Geometry: final body of the model. Coordinates: model frame, mm. A direction names the side the tool comes from. Coordinates: 2 decimals unless noted, no trailing zeros. Loops run counter-clockwise (first coordinate to the right, second up) from the corner with the lowest first, then second, coordinate; pieces in that order, holes last. Notation, with made-up numbers: (87, 8) - (98, 8) arc R16 ccw to (98, 16) - close; hole circle Ø11 at (70.5, 55.5). An arc over 180 degrees is marked (long way). Return JSON: item names as keys, results as strings.
from build123d import *

# Parameters (mm, degrees)
SKETCH10_W                   = 276.86
SKETCH10_H                   = 12.7
BASE_FLANGE1_DEPTH           = 1
EDGE_FLANGE1_STRIP_W         = 9.08
EDGE_FLANGE1_STRIP_H         = 1
EDGE_FLANGE1_STRIP_CUT_DEPTH = 276.86
EDGE_FLANGE1_DEPTH           = 276.86
EDGE_FLANGE2_STRIP_W         = 9.08
EDGE_FLANGE2_STRIP_H         = 1
EDGE_FLANGE2_STRIP_CUT_DEPTH = 276.86
EDGE_FLANGE2_DEPTH           = 276.86
EDGE_FLANGE3_STRIP_W         = 9.08
EDGE_FLANGE3_STRIP_H         = 1
EDGE_FLANGE3_STRIP_CUT_DEPTH = 5.62
EDGE_FLANGE3_DEPTH           = 5.62


# Sheet-metal steps are written as plain solids
with BuildPart() as part:
    # Sketch10 → Base-Flange1 (new body)
    with BuildSketch(Plane(origin=(0, 0, 0), x_dir=(1, 0, 0), z_dir=(0, 1, 0))):
        Rectangle(SKETCH10_W, SKETCH10_H)
    extrude(amount=-BASE_FLANGE1_DEPTH)

    # Edge-Flange1 strip (across the edge) → Edge-Flange1 strip cut (cut)
    with BuildSketch(Plane(origin=(138.43, 0, -6.35), x_dir=(0, 0, 1), z_dir=(-1, 0, 0))):
        with Locations((-1, -0.5)):
            Rectangle(EDGE_FLANGE1_STRIP_W, EDGE_FLANGE1_STRIP_H)
    extrude(amount=EDGE_FLANGE1_STRIP_CUT_DEPTH, mode=Mode.SUBTRACT)

    # Edge-Flange1 section (across the edge) → Edge-Flange1 (add)
    with BuildSketch(Plane(origin=(138.43, 0, -6.35), x_dir=(0, 0, 1), z_dir=(-1, 0, 0))):
        with BuildLine():
            Line((0, 2.54), (0, 11.7))
            Line((0, 11.7), (1, 11.7))
            Line((1, 11.7), (1, 2.54))
            ThreePointArc((1, 2.54), (1.743948776, 0.743948776), (3.54, 0))
            Line((3.54, 0), (3.54, -1))
            ThreePointArc((3.54, -1), (1.036841995, 0.036841995), (0, 2.54))
        make_face()
    extrude(amount=EDGE_FLANGE1_DEPTH)

    # Edge-Flange2 strip (across the edge) → Edge-Flange2 strip cut (cut)
    with BuildSketch(Plane(origin=(-138.43, 0, 6.35), x_dir=(0, 0, -1), z_dir=(1, 0, 0))):
        with Locations((-1, -0.5)):
            Rectangle(EDGE_FLANGE2_STRIP_W, EDGE_FLANGE2_STRIP_H)
    extrude(amount=EDGE_FLANGE2_STRIP_CUT_DEPTH, mode=Mode.SUBTRACT)

    # Edge-Flange2 section (across the edge) → Edge-Flange2 (add)
    with BuildSketch(Plane(origin=(-138.43, 0, 6.35), x_dir=(0, 0, -1), z_dir=(1, 0, 0))):
        with BuildLine():
            Line((0, 2.54), (0, 11.7))
            Line((0, 11.7), (1, 11.7))
            Line((1, 11.7), (1, 2.54))
            ThreePointArc((1, 2.54), (1.743948776, 0.743948776), (3.54, 0))
            Line((3.54, 0), (3.54, -1))
            ThreePointArc((3.54, -1), (1.036841995, 0.036841995), (0, 2.54))
        make_face()
    extrude(amount=EDGE_FLANGE2_DEPTH)

    # Edge-Flange3 strip (across the edge) → Edge-Flange3 strip cut (cut)
    with BuildSketch(Plane(origin=(-138.43, 0, -2.81), x_dir=(1, 0, 0), z_dir=(0, 0, 1))):
        with Locations((-1, -0.5)):
            Rectangle(EDGE_FLANGE3_STRIP_W, EDGE_FLANGE3_STRIP_H)
    extrude(amount=EDGE_FLANGE3_STRIP_CUT_DEPTH, mode=Mode.SUBTRACT)

    # Edge-Flange3 section (across the edge) → Edge-Flange3 (add)
    with BuildSketch(Plane(origin=(-138.43, 0, -2.81), x_dir=(1, 0, 0), z_dir=(0, 0, 1))):
        with BuildLine():
            Line((0, 2.54), (0, 11.7))
            Line((0, 11.7), (1, 11.7))
            Line((1, 11.7), (1, 2.54))
            ThreePointArc((1, 2.54), (1.743948776, 0.743948776), (3.54, 0))
            Line((3.54, 0), (3.54, -1))
            ThreePointArc((3.54, -1), (1.036841995, 0.036841995), (0, 2.54))
        make_face()
    extrude(amount=EDGE_FLANGE3_DEPTH)


solid = part.part
Item 1: Mould query, pull axis Z, two halves, no side actions, for faces 1 (the face through (-2, 7, 6.35)), 2 (the face through (-2, 7, 5.35)), 3 (the face through (0, -1, 0)). Classes: +Z half, -Z half, draft (parallel to the pull), parting line (faces both ways), or undercut.
Worked out:
{"face 1": "+Z half", "face 2": "undercut", "face 3": "draft"}
Item 2: Section query B-B, the plane x = 20. Return loops of the section in (y, z), and give its area (3 significant figures).
Worked out:
{"outline": "(-1, -2.81) arc R3.54 ccw to (2.54, -6.35) - (11.7, -6.35) - (11.7, -5.35) - (2.54, -5.35) arc R2.54 cw to (0, -2.81) - (0, 2.81) arc R2.54 cw to (2.54, 5.35) - (11.7, 5.35) - (11.7, 6.35) - (2.54, 6.35) arc R3.54 ccw to (-1, 2.81) - close", "area": "33.5 mm^2"}
Item 3: Reachability of faces 4 (the face through (2, 7, -5.35)), 5 (the face through (-137.43, 7, 0)), 6 (the face through (2, 7, -6.35)) from +Z, -Z, +X, -X, +Y, -Y: full face, straight path, thin tool, end or side. Return the list, or none.
Worked out:
{"face 4": "+X, -X, +Y", "face 5": "+X, +Y", "face 6": "-Z, +X, -X, +Y, -Y"}
Item 4: Section query A-A, the plane y = 7.25. Return loops of the section in (x, z), and give its area (3 significant figures).
Worked out:
{"outline": "(-138.43, -6.35) - (138.43, -6.35) - (138.43, -5.35) - (-138.43, -5.35) - close; (-138.43, -2.81) - (-137.43, -2.81) - (-137.43, 2.81) - (-138.43, 2.81) - close; (-138.43, 5.35) - (138.43, 5.35) - (138.43, 6.35) - (-138.43, 6.35) - close", "area": "559 mm^2"}
Item 5: First-contact query: pin 1 Ø3 at (x, z) = (18, 1.5) entering from +Y; pin 2 Ø2 at (y, z) = (5.5, 0.5) entering from +X; pin 3 Ø0.8 at (x, y) = (-136, -0.5) entering from +Z. Flat tips, straight axial feed; report the tip coordinate or a pass-through.
Worked out:
{"pin 1": "y = 0.01", "pin 2": "x = -137.43", "pin 3": "z = 5.17"}
Item 6: Ray query, probe 1 along Z at (x, y) = (105, 9); probe 2 along Y at (x, z) = (44, 2.25); probe 3 along Z at (x, y) = (39, 1). Return the intervals inside material, ascending. Write a range as from..to.
Worked out:
{"probe 1": "-6.35..-5.35, 5.35..6.35", "probe 2": "-1..0", "probe 3": "-6..-4.83, 4.83..6"}
